```python
from build123d import *

# Parameters (mm, degrees)
BOSS_EXTRUDE2_DEPTH = 10
BOSS_EXTRUDE3_DEPTH = 4
CUT_EXTRUDE1_DEPTH  = 4
SKETCH7_R           = 1
CUT_EXTRUDE2_DEPTH  = 11
SKETCH9_W           = 12.5
SKETCH9_H           = 3.55
CUT_EXTRUDE7_DEPTH  = 12.800523878
SKETCH11_R          = 1.5
CUT_EXTRUDE8_DEPTH  = 15


with BuildPart() as part:
    # Sketch1 → Boss-Extrude2 (new body)
    with BuildSketch(Plane(origin=(0, 0, 0), x_dir=(1, 0, 0), z_dir=(0, 1, 0))):
        with BuildLine():
            Line((19.837809991, 13.8), (19.837809991, 1.999476122))
            Line((19.837809991, 1.999476122), (42.1, 1.999476122))
            ThreePointArc((42.1, 1.999476122), (48.000261939, 7.899738061), (42.1, 13.8))
            Line((42.1, 13.8), (19.837809991, 13.8))
        make_face()
    extrude(amount=BOSS_EXTRUDE2_DEPTH)

    # Sketch4 → Boss-Extrude3 (add)
    with BuildSketch(Plane(origin=(0, 0, 0), x_dir=(-1, 0, 0), z_dir=(0, -1, 0))):
        with BuildLine():
            Line((-19.837809991, 2), (-19.837809991, 13.8))
            Line((-19.837809991, 13.8), (-42.1, 13.8))
            ThreePointArc((-42.1, 13.8), (-48, 7.9), (-42.1, 2))
            Line((-42.1, 2), (-19.837809991, 2))
        make_face()
    extrude(amount=BOSS_EXTRUDE3_DEPTH)

    # Sketch6 → Cut-Extrude1 (cut)
    with BuildSketch(Plane.XZ.offset(4)):
        with BuildLine():
            Line((28.779938833, -2.819139544), (40.580172538, -4.504631907))
            ThreePointArc((40.580172538, -4.504631907), (45.727347719, -8.725074859), (39.261067618, -10.303926565))
            Line((39.261067618, -10.303926565), (27.892761565, -6.719513435))
            ThreePointArc((27.892761565, -6.719513435), (26.386163253, -4.325737856), (28.779938833, -2.819139544))
        make_face()
    extrude(amount=-CUT_EXTRUDE1_DEPTH, mode=Mode.SUBTRACT)

    # Sketch7 → Cut-Extrude2 (cut, through all)
    with BuildSketch(Plane.XZ):
        with Locations((42.1, -7.9)):
            Circle(SKETCH7_R)
    extrude(amount=-CUT_EXTRUDE2_DEPTH, mode=Mode.SUBTRACT)

    # Sketch9 → Cut-Extrude7 (cut, through all)
    with BuildSketch(Plane.XY.offset(-1.999476122)):
        with Locations((26.087809991, 5)):
            Rectangle(SKETCH9_W, SKETCH9_H)
    extrude(amount=-CUT_EXTRUDE7_DEPTH, mode=Mode.SUBTRACT)

    # Sketch11 → Cut-Extrude8 (cut, through all)
    with BuildSketch(Plane(origin=(0, 10, 0), x_dir=(1, 0, 0), z_dir=(0, 1, 0))):
        with Locations((30.53490887, 9.85)):
            Circle(SKETCH11_R)
        with Locations((26.53490887, 9.85)):
            Circle(SKETCH11_R)
        with Locations((22.53490887, 9.85)):
            Circle(SKETCH11_R)
    extrude(amount=-CUT_EXTRUDE8_DEPTH, mode=Mode.SUBTRACT)


solid = part.part
```
Here's how the part is built. I have some questions about the finished solid (model axes, mm). A direction names the side the tool comes from. Round coordinates to 2 decimals unless told otherwise and drop trailing zeros. Order: outer loops, then holes, each group sorted by start corner. A loop starts at its lowest first (then second) coordinate and runs counter-clockwise, first axis right, second up. Notation, with made-up numbers: M 30.5,-12 L 51.5,-12 A13 ccw 51.5,3 Z; hole C 50,22.5 d11. An arc over 180 degrees is marked long. Answer as CSV lines item,"result".
Item 1: We'd pull the mould along Z, two halves only. Please class faces 4 (the flat face through (26, 3.225, -8)), 5 (the cylindrical face through (29.036, 8.41, -9.916)), 6 (the flat face through (31, 3, -13.8)), 7 (the cylindrical face through (22.34, -0.337, -11.337)): +Z half, -Z half, draft (parallel to the pull), parting line (faces both ways), or undercut.
From the geometry:
face 4,"draft"
face 5,"undercut"
face 6,"-Z half"
face 7,"undercut"
Item 2: Please list where these lines run through material, in increasing order: L1, parallel to Y at x = 25, z = -9.5 (3 decimals); L2, parallel to Z at x = 42.1, y = -1.9; L3, parallel to Z at x = 42.1, y = 4.25. Write a range as [from, to].
From the geometry:
L1,"[-4, 3.225], [6.775, 10]"
L2,"[-13.8, -11.62], [-4.18, -2]"
L3,"[-13.8, -8.9], [-6.9, -2]"
Item 3: For pin 1 (1.8 mm diameter, centred on y = 4.5, z = -7.5, fed in from -X); pin 2 (1.6 mm diameter, centred on x = 42.1, z = -7.9, fed in from -Y); pin 3 (3.5 mm diameter, centred on x = 39.5, z = -8.5, fed in from -Y), each with a flat end and sliding along its axis, tell me the tip position at first contact or that it passes through.
From the geometry:
pin 1,"x = 32.34"
pin 2,"through"
pin 3,"y = 0"
Item 4: Imagine slicing it at A-A on y = 2.25. List the corners of the cut face in (x, z) for me, and give its area (3 significant figures).
From the geometry:
outline,"M 19.84,-13.8 L 42.1,-13.8 A5.9 ccw 42.1,-2 L 19.84,-2 Z; hole C 22.53,-9.85 d3; hole C 26.53,-9.85 d3; hole C 30.53,-9.85 d3; hole C 42.1,-7.9 d2"
area,"293 mm2"
Item 5: Imagine slicing it at B-B on y = 4.75. List the corners of the cut face in (x, z) for me.
From the geometry:
outline,"M 32.34,-13.8 L 42.1,-13.8 A5.9 ccw 42.1,-2 L 32.34,-2 Z; hole C 42.1,-7.9 d2"
Item 6: Which directions (+Z, -Z, +X, -X, +Y, -Y) give clear straight access to the entire face, cutting with the end or side of a thin tool? Please do faces 1 (the flat face through (32.338, 5, -8)), 2 (the cylindrical face through (48, -2, -8)), 3 (the flat face through (36, 0, -7)).
From the geometry:
face 1,"+Z, -Z, -X"
face 2,"+X, +Y, -Y"
face 3,"-Y"
